```python
from build123d import *

# Parameters (mm, degrees)
RESSALTO_EXTRUS_O1_OUTLINE_R = 1.499997
RESSALTO_EXTRUS_O1_DEPTH     = 30
ESBO_O2_R                    = 1.5
CORTE_EXTRUS_O1_DEPTH        = 30


# Read off the part's stored shape, not the designer's step: Ressalto-extrusão1
with BuildPart() as part:
    # Ressalto-extrusão1 outline → Ressalto-extrusão1 (new body)
    with BuildSketch(Plane.XY):
        Polygon((-5.588, -17.863), (-5.588, -6.814), (5.588, -6.814), (5.588, -17.736), (5.646801, -18.1358468), (5.8082688, -18.4582998), (6.0501022, -18.6736156), (6.1941964, -18.7317816), (6.35, -18.752), (6.5058036, -18.7317816), (6.6498978, -18.6736156), (6.8917312, -18.4582998), (7.053199, -18.1358468), (7.112, -17.736), (7.112, -6.814), (12.192, -6.814), (12.192, -17.736), (12.250801, -18.1358468), (12.4122688, -18.4582998), (12.6541022, -18.6736156), (12.7981964, -18.7317816), (12.954, -18.752), (13.1098036, -18.7317816), (13.2538978, -18.6736156), (13.4957312, -18.4582998), (13.657199, -18.1358468), (13.716, -17.736), (13.716, -2.75), (-13.716, -2.75), (-13.716, -17.736), (-13.657199, -18.1358468), (-13.4957312, -18.4582998), (-13.2538978, -18.6736156), (-13.1098036, -18.7317816), (-12.954, -18.752), (-12.7981964, -18.7317816), (-12.6541022, -18.6736156), (-12.4122688, -18.4582998), (-12.250801, -18.1358468), (-12.192, -17.736), (-12.192, -6.814), (-7.112, -6.814), (-7.112, -17.863), (-7.053199, -18.2628468), (-6.8917312, -18.5852998), (-6.6498978, -18.8006156), (-6.5058036, -18.8587816), (-6.35, -18.879), (-6.1941964, -18.8587816), (-6.0501022, -18.8006156), (-5.8082688, -18.5852998), (-5.646801, -18.2628468), align=None)
        with Locations((-7.9375, -5.29)):
            Circle(RESSALTO_EXTRUS_O1_OUTLINE_R, mode=Mode.SUBTRACT)
        with Locations((7.9375, -5.29)):
            Circle(RESSALTO_EXTRUS_O1_OUTLINE_R, mode=Mode.SUBTRACT)
    extrude(amount=RESSALTO_EXTRUS_O1_DEPTH)

    # Esboço2 → Corte-extrusão1 (cut)
    with BuildSketch(Plane(origin=(0, -2.75, 0), x_dir=(1, 0, 0), z_dir=(0, 1, 0))):
        with Locations(Location((0.635, -20, 0), (0, 0, 270))):
            Circle(ESBO_O2_R)
    extrude(amount=-CORTE_EXTRUS_O1_DEPTH, mode=Mode.SUBTRACT)


solid = part.part
```
Read the model definition and answer for the solid it produces. Units are mm, in the model's axes. A direction names the side the tool comes from. Coordinates: 2 decimals unless noted, no trailing zeros. Write each loop counter-clockwise with the first axis right and the second up, starting at its lowest first coordinate (ties: lowest second). Pieces come first, ordered by that corner, then holes. Notation, with made-up numbers: (-29.5, 75.5) - (10.5, 75.5) arc R24 cw to (10.5, 100.5) - close; hole circle Ø9 at (66, 29). An arc over 180 degrees is marked (long way). Answer as a JSON object with one key per item and string values. Group by question number.
1. A cutting plane is placed at D-D (x = 5). Determine the outline of the cut face in (y, z), plus the area to 3 significant figures.
2. Each of these flat-tipped pins is pushed along its axis until it touches: P1, Ø3.5, axis at x = 2.5, z = 22.5, coming from the -Y side; P2, Ø1, axis at x = -4.5, y = -15.5, coming from the -Z side. Where does it stop, or does it pass through?
3. A cutting plane is placed at A-A (y = -6.25). Determine the outline of the cut face in (x, z) (3 decimals), plus the area to 3 significant figures.
4. Consider L1, parallel to X at y = -11.25, z = 11.5; L2, parallel to X at y = -6.25, z = 9; L3, parallel to X at y = -5.9, z = 20 (3 decimals). Determine where each line is inside the solid, lowest interval first. Write a range as [from, to].
5. The mould has two halves that part along X. Classify faces 1 (the flat face through (12.192, -12, 15)), 2 (the flat face through (-3, -5, 0)), 3 (the flat face through (-13.716, -10, 15)), 4 (the flat face through (13.716, -10, 15)): +X half, -X half, draft (parallel to the pull), parting line (faces both ways), or undercut.
6. Which of the six approach directions +Z, -Z, +X, -X, +Y, -Y give full straight-line access (tool end or side, diameter ignored) to faces 5 (the cylindrical face through (6.44, -5.22, 14.79)), 6 (the flat face through (-10, -6.814, 15))?
7. A cutting plane is placed at B-B (y = -8.25). Determine the outline of the cut face in (x, z), plus the area to 3 significant figures.
8. A cutting plane is placed at C-C (z = 20). Give the number of separate pieces and of enclosed holes in the cut face, plus the area to 3 significant figures.
Worked out:
{
 "1": {"outline": "(-6.81, 0) - (-2.75, 0) - (-2.75, 30) - (-6.81, 30) - close", "area": "122 mm²"},
 "2": {"P1": "stops at y = -6.81", "P2": "passes through"},
 "3": {"outline": "(-13.716, 0) - (-9.09, 0) - (-9.09, 30) - (-13.716, 30) - close; (-6.785, 0) - (6.785, 0) - (6.785, 30) - (-6.785, 30) - close; (9.09, 0) - (13.716, 0) - (13.716, 30) - (9.09, 30) - close; hole circle Ø3 at (0.635, 20)", "area": "678 mm²"},
 "4": {"L1": "x = [-13.72, -12.19], [-7.11, -5.59], [5.59, 7.11], [12.19, 13.72]", "L2": "x = [-13.72, -9.09], [-6.78, 6.78], [9.09, 13.72]", "L3": "x = [-13.716, -9.308], [-6.567, -0.865], [2.135, 6.567], [9.308, 13.716]"},
 "5": {"face 1": "undercut", "face 2": "draft", "face 3": "-X half", "face 4": "+X half"},
 "6": {"face 5": "+Z, -Z", "face 6": "+Z, -Z, -Y"},
 "7": {"outline": "(-13.72, 0) - (-12.19, 0) - (-12.19, 30) - (-13.72, 30) - close; (-7.11, 0) - (-5.59, 0) - (-5.59, 30) - (-7.11, 30) - close; (5.59, 0) - (7.11, 0) - (7.11, 30) - (5.59, 30) - close; (12.19, 0) - (13.72, 0) - (13.72, 30) - (12.19, 30) - close", "area": "183 mm²"},
 "8": {"separate pieces": "2", "enclosed holes": "2", "area": "157 mm²"}
}
